Geometry check sheet. Reference: the model listing, model coordinates, mm. A direction names the side the tool comes from. Round coordinates to 2 decimals unless told otherwise and drop trailing zeros. Order: outer loops, then holes, each group sorted by start corner. A loop starts at its lowest first (then second) coordinate and runs counter-clockwise, first axis right, second up.
(1) Cross-section at C-C on z = 9. Enter the section's corners in (x, y), and give its area (3 significant figures).
(2) Gauge pin test, flat ends, axial feed: P1, Ø1.5, axis at y = 4, z = 0.5, coming from the -X side; P2, Ø12, axis at x = -13.5, z = 9.5, coming from the -Y side; P3, Ø2, axis at y = 4, z = -2, coming from the -X side. Record the tip position at first contact, or that the pin passes through.
(3) Cross-section at D-D on z = 18. Enter the section's corners in (x, y), and give its area (3 significant figures).
(4) Cross-section at B-B on x = -16.5. Enter the section's corners in (y, z).
(5) Cross-section at A-A on y = 1.4. Enter the section's corners in (x, z).
(6) Set-up check for faces 1 (the face through (-48.11, 2.46, -15.5)), 2 (the face through (68.262, 2, 23)), 3 (the face through (43.327, 2.465, -15.334)), 4 (the face through (-5, 1, 20)), 5 (the face through (1, 5, 17)): record each of +Z, -Z, +X, -X, +Y, -Y from which the full face is reachable in a straight line by a thin tool's end or side.
(7) Draft check along X on faces 6 (the face through (-30.26, 1.48, 0.32)), 7 (the face through (43.971, 2.465, 15.637)), 8 (the face through (1, 0, 23)). Enter one of: pulls with the +X half, pulls with the -X half, needs draft (parallel to the pull), parting line crosses it, or undercut.
(8) Thickness scan on L1, parallel to Z at x = -5.5, y = 4.75; L2, parallel to Z at x = -7.5, y = 1.65; L3, parallel to X at y = 2.2, z = 16. Record the ranges inside material, lowest first.
Autodesk Inventor part; units mm, degrees
ref_plane "YZ Plane" through (0, 0, 0) normal (1, 0, 0) x (0, 1, 0)
ref_plane "XZ Plane" through (0, 0, 0) normal (0, 1, 0) x (-1, 0, 0)
ref_plane "XY Plane" through (0, 0, 0) normal (0, 0, 1) x (1, 0, 0)
sketch "Sketch1" plane through (0, 0, 0) normal (0, 1, 0) x (-1, 0, 0)
  line L0 (-68.2625, -25) -> (68.2625, -25)
  line L1 (68.2625, -25) -> (68.2625, 25)
  line L2 (68.2625, 25) -> (-68.2625, 25)
  line L3 (-68.2625, 25) -> (-68.2625, -25)
  line L4 (-68.2625, -25) -> (68.2625, 25) construction
  line L5 (68.2625, -25) -> (-68.2625, 25) construction
  point P0 (0, 0)
  dimension "d0" = 136.525
  dimension "d1" = 50
extrude "Extrusion1" add sketch "Sketch1" along normal blind 5
sketch "Sketch2" plane through (0, 0, 0) normal (0, -1, 0) x (1, 0, 0)
  circle A0 centre (-4.7625, 0) radius 25.5
  line L0 (-68.2625, -25) -> (-68.2625, 25)
  line L1 (-20.5818, -20) -> (11.0568, -20)
  line L2 (-20.5818, 20) -> (11.0568, 20)
  point P0 (0, 0)
  dimension "d4" = 51
  dimension "d5" = 63.5
  dimension "d6" = 40
  dimension "d7" = 20
extrude "Extrusion2" cut sketch "Sketch2" against normal blind 3 contours A0 L1 L2
sketch "Sketch3" plane through (0, 0, 0) normal (0, -1, 0) x (1, 0, 0)
  line L0 (68.2625, 25) -> (68.2625, -25)
  arc A0 (23.7375, 0) -> (68.2625, -21) centre (68.2625, 36.7018) ccw
  arc A1 (68.2625, 21) -> (23.7375, 0) centre (68.2625, -36.7018) ccw
  arc A2 (11.0568, -20) -> (11.0568, 20) centre (-4.7625, 0) ccw
  line L1 (-68.2625, -25) -> (-68.2625, 25)
  arc A3 (-68.2625, -21) -> (-33.2625, 0) centre (-68.2625, 18.6667) ccw
  arc A4 (-33.2625, 0) -> (-68.2625, 21) centre (-68.2625, -18.6667) ccw
  arc A5 (-20.5818, 20) -> (-20.5818, -20) centre (-4.7625, 0) ccw
  line L2 (10.2375, 15) -> (-19.7625, 15)
  line L3 (-19.7625, 15) -> (-19.7625, -15)
  line L4 (-19.7625, -15) -> (10.2375, -15)
  line L5 (10.2375, -15) -> (10.2375, 15)
  line L6 (10.2375, 15) -> (-19.7625, -15) construction
  line L7 (-19.7625, 15) -> (10.2375, -15) construction
  point P0 (0, 0)
  point P1 (20.7375, 0)
  point P2 (-30.2625, 0)
  dimension "d10" = 4
  dimension "d11" = 4
  dimension "d12" = 3
  dimension "d13" = 4
  dimension "d14" = 4
  dimension "d15" = 3
  dimension "d16" = 30
  dimension "d17" = 30
extrude "Extrusion3" cut sketch "Sketch3" against normal through all
equation "\"d11\" = d10"
equation "\"d14\" = d13"
properties part number "Spin Arrest"
Found:
1. outline: (-39.84, 0) - (-28.62, 0) - (-28.62, 3) - (-19.76, 3) - (-19.76, 5) - (-39.84, 5) - close; (10.24, 3) - (19.1, 3) - (19.1, 0) - (33.04, 0) - (33.04, 5) - (10.24, 5) - close
1. area: 161 mm2
2. P1: stops at x = -33.96
2. P2: stops at y = 3
2. P3: stops at x = -35.04
3. outline: (-53.13, 0) - (-22.82, 0) - (-22.82, 3) - (13.3, 3) - (13.3, 0) - (49.9, 0) - (49.9, 5) - (-53.13, 5) - close
3. area: 407 mm2
4. outline: (0, -25) - (5, -25) - (5, -15) - (3, -15) - (3, -20) - (0, -20) - close; (0, 20) - (3, 20) - (3, 15) - (5, 15) - (5, 25) - (0, 25) - close
5. outline: (-68.26, -25) - (68.26, -25) - (68.26, -21) arc R57.7 cw to (23.74, 0) arc R57.7 cw to (68.26, 21) - (68.26, 25) - (-68.26, 25) - (-68.26, 21) arc R39.67 cw to (-33.26, 0) arc R39.67 cw to (-68.26, -21) - close; hole (-20.58, -20) - (11.06, -20) arc R25.5 ccw to (11.06, 20) - (-20.58, 20) arc R25.5 ccw to start
6. face 1: -X, +Y, -Y
6. face 2: +Z, -Z, +X, +Y, -Y
6. face 3: +X, +Y, -Y
6. face 4: -Y
6. face 5: +Z, -Z, +X, -X, +Y
7. face 6: undercut
7. face 7: pulls with the +X half
7. face 8: needs draft
8. L1: z = -25 to -15, 15 to 25
8. L2: z = -25 to -20, 20 to 25
8. L3: x = -48.98 to -24.62, 15.09 to 44.77
